from build123d import *

# Parameters (mm, degrees)
F0_W      = 18
F0_H      = 12
F1_DEPTH  = 1.5
F2_W      = 14
F2_H      = 10
F3_DEPTH  = 20
F4_W      = 3
F4_H      = 20
F5_DEPTH  = 25
F7_D      = 4.2
F8_W      = 10.9
F8_H      = 2.4
F9_DEPTH  = 2.5
F10_W     = 10.9
F10_H     = 2.75
F10_H_2   = 2.4
F11_DEPTH = 1.5


with BuildPart() as f1:
    # F0 (on Top) → F1 (new body, symmetric)
    with BuildSketch(Plane.XY):
        Rectangle(F0_W, F0_H)
    extrude(amount=F1_DEPTH, both=True)

    # F2 (on face) → F3 (join)
    with BuildSketch(Plane.XY.offset(1.5)):
        Rectangle(F2_W, F2_H)
    extrude(amount=F3_DEPTH)

    # F4 (on face) → F5 (cut)
    with BuildSketch(Plane.YZ.offset(7)):
        with Locations((0, 11.5)):
            Rectangle(F4_W, F4_H)
    extrude(amount=-F5_DEPTH, mode=Mode.SUBTRACT)

    # F7 (through all)
    with Locations(Plane.XZ.offset(5)):
        with Locations((0, 18.5)):
            Hole(F7_D / 2)

    # F8 (on face) → F9 (join)
    with BuildSketch(Plane(origin=(0, 0, -1.5), x_dir=(1, 0, 0), z_dir=(0, 0, -1))):
        Rectangle(F8_W, F8_H)
    extrude(amount=F9_DEPTH)

    # F10 (on face) → F11 (join)
    with BuildSketch(Plane(origin=(0, 0, -4), x_dir=(1, 0, 0), z_dir=(0, 0, -1))):
        with Locations((0, -2.575)):
            Rectangle(F10_W, F10_H)
        Rectangle(F10_W, F10_H_2)
        with Locations((0, 2.575)):
            Rectangle(F10_W, F10_H)
    extrude(amount=F11_DEPTH)


solid = f1.part
The listing builds one solid part. Answer for the finished solid, in the listing's coordinates (mm). A direction names the side the tool comes from. Give positions to 0.01 mm unless a question says otherwise; leave off trailing zeros. Loops run counter-clockwise (first coordinate to the right, second up) from the corner with the lowest first, then second, coordinate; pieces in that order, holes last. Notation, with made-up numbers: M 64.5,12.5 L 96.5,12.5 A19 cw 96.5,22.5 Z; hole C -39,16 d6. An arc over 180 degrees is marked long. Answer as CSV lines item,"result".
Item 1: Straight lines are drawn through the part: line 1 along Z through (x, y) = (0, -2.8); line 2 along Z through (x, y) = (4, -2); line 3 along Y through (x, z) = (1.5, 12). For each, find the intervals that lie inside material, in ascending order. Write a range as [from, to].
Values follow:
line 1,"z = [-5.5, -4], [-1.5, 16.4], [20.6, 21.5]"
line 2,"z = [-5.5, -4], [-1.5, 21.5]"
line 3,"y = [-5, -1.5], [1.5, 5]"
Item 2: The part is cut by section B-B (z = 18.5). Give the vertices of the cut face in (x, y).
Values follow:
outline,"M -7,-5 L -2.1,-5 L -2.1,-1.5 L -7,-1.5 Z; M -7,1.5 L -2.1,1.5 L -2.1,5 L -7,5 Z; M 2.1,-5 L 7,-5 L 7,-1.5 L 2.1,-1.5 Z; M 2.1,1.5 L 7,1.5 L 7,5 L 2.1,5 Z"
Item 3: Given pin 1 Ø2.5 at (x, z) = (0, 18.5) entering from +Y; pin 2 Ø7 at (x, z) = (-3, 12.5) entering from -Y; pin 3 Ø1.8 at (y, z) = (4, 6.5) entering from +X; pin 4 Ø5 at (x, z) = (5.5, 16.5) entering from +Y, each flat-ended and moving along its own axis, determine where each tip first touches the part or whether it passes through.
Values follow:
pin 1,"passes through"
pin 2,"stops at y = -5"
pin 3,"stops at x = 7"
pin 4,"stops at y = 5"
Item 4: The part is cut by section A-A (y = -3). Give the vertices of the cut face in (x, z).
Values follow:
outline,"M -9,-1.5 L 9,-1.5 L 9,1.5 L 7,1.5 L 7,21.5 L -7,21.5 L -7,1.5 L -9,1.5 Z; M -5.45,-5.5 L 5.45,-5.5 L 5.45,-4 L -5.45,-4 Z; hole C 0,18.5 d4.2"
Item 5: The part is cut by section C-C (x = 0). Give the vertices of the cut face in (y, z).
Values follow:
outline,"M -6,-1.5 L -1.2,-1.5 L -1.2,-4 L -3.95,-4 L -3.95,-5.5 L 3.95,-5.5 L 3.95,-4 L 1.2,-4 L 1.2,-1.5 L 6,-1.5 L 6,1.5 L 5,1.5 L 5,16.4 L 1.5,16.4 L 1.5,1.5 L -1.5,1.5 L -1.5,16.4 L -5,16.4 L -5,1.5 L -6,1.5 Z; M -5,20.6 L -1.5,20.6 L -1.5,21.5 L -5,21.5 Z; M 1.5,20.6 L 5,20.6 L 5,21.5 L 1.5,21.5 Z"
Item 6: Which of the six approach directions +Z, -Z, +X, -X, +Y, -Y give full straight-line access (tool end or side, diameter ignored) to faces 5 (the flat face through (0, 3.95, -5)), 6 (the flat face through (-7, 3, 11)), 7 (the flat face through (5.45, 0, -4)), 8 (the flat face through (7, -3, 11)), 9 (the flat face through (0, 5, 11))?
Values follow:
face 5,"-Z, +X, -X, +Y"
face 6,"+Z, -X, +Y, -Y"
face 7,"-Z, +X, +Y, -Y"
face 8,"+Z, +X, +Y, -Y"
face 9,"+Z, +X, -X, +Y"
Item 7: The mould has two halves that part along Z. Classify faces 1 (the flat face through (7, 3, 11)), 2 (the flat face through (0, 1.2, -3)), 3 (the flat face through (0, 0, -5.5)), 4 (the flat face through (0, -3, -4)): released by +Z, released by -Z, zero draft, split by the parting line, or undercut.
Values follow:
face 1,"zero draft"
face 2,"undercut"
face 3,"released by -Z"
face 4,"undercut"
Item 8: The part is cut by section D-D (x = -6.25). Give the vertices of the cut face in (y, z).
Values follow:
outline,"M -6,-1.5 L 6,-1.5 L 6,1.5 L 5,1.5 L 5,21.5 L 1.5,21.5 L 1.5,1.5 L -1.5,1.5 L -1.5,21.5 L -5,21.5 L -5,1.5 L -6,1.5 Z"
